```python
from build123d import *

# Parameters (mm, degrees)
SKETCH1_R                       = 62.5
SKETCH1_R_2                     = 36
BOSS_EXTRUDE1_DEPTH             = 5
SKETCH1_4_R                     = 51.5
SKETCH1_4_R_2                   = 36
BOSS_EXTRUDE2_DEPTH             = 14.5
F_4_0MM_DOWEL_HOLE3_D           = 4
F_4_0MM_DOWEL_HOLE3_CSINK_D     = 4.05
F_4_0MM_DOWEL_HOLE3_CSINK_ANGLE = 90
SKETCH11_R                      = 47.5
CUT_EXTRUDE4_DEPTH              = 10.5
FILLET1_R                       = 1


with BuildPart() as part:
    # Sketch1 → Boss-Extrude1 (new body)
    with BuildSketch(Plane.XY):
        Circle(SKETCH1_R)
        Circle(SKETCH1_R_2, mode=Mode.SUBTRACT)
    extrude(amount=BOSS_EXTRUDE1_DEPTH)

    # Sketch1_4 → Boss-Extrude2 (add)
    with BuildSketch(Plane.XY):
        with Locations(Location((0, 0, 0), (0, 0, 180))):
            Circle(SKETCH1_4_R)
        Circle(SKETCH1_4_R_2, mode=Mode.SUBTRACT)
    extrude(amount=BOSS_EXTRUDE2_DEPTH)

    # 4.0mm Dowel Hole3 (through all)
    with Locations(Plane(origin=(0, 0, 0), x_dir=(-1, 0, 0), z_dir=(0, 0, -1))):
        with Locations((0, 57), (0, 42), (40.305086528, 40.305086528), (29.69848481, 29.69848481), (42, 0), (57, 0), (40.305086528, -40.305086528), (29.69848481, -29.69848481), (0, -42), (0, -57), (-29.69848481, -29.69848481), (-40.305086528, -40.305086528), (-42, 0), (-57, 0), (-29.69848481, 29.69848481), (-40.305086528, 40.305086528)):
            CounterSinkHole(F_4_0MM_DOWEL_HOLE3_D / 2, F_4_0MM_DOWEL_HOLE3_CSINK_D / 2, counter_sink_angle=F_4_0MM_DOWEL_HOLE3_CSINK_ANGLE)

    # Sketch11 → Cut-Extrude4 (cut)
    with BuildSketch(Plane.XY):
        with Locations(Location((0, 0, 0), (0, 0, 180))):
            Circle(SKETCH11_R)
    extrude(amount=CUT_EXTRUDE4_DEPTH, mode=Mode.SUBTRACT)

    # Fillet1
    fillet1_edges = [part.edges().sort_by_distance(p)[0] for p in [
        (51.5, 0, 5),
        (51.5, 0, 14.5),
        (47.5, 0, 10.5),
    ]]
    fillet(fillet1_edges, radius=FILLET1_R)


solid = part.part
```
The listing builds one solid part. Answer for the finished solid, in the listing's coordinates (mm). A direction names the side the tool comes from. Round coordinates to 2 decimals unless told otherwise and drop trailing zeros. Loops run counter-clockwise (first coordinate to the right, second up) from the corner with the lowest first, then second, coordinate; pieces in that order, holes last.
Q1. Section A-A, the plane x = 57 is taken. Determine the outline of the cut face in (y, z) (3 decimals), then the cut area to 3 significant figures.
Q2. For a pull along X with two mould halves and no side action, classify faces 1 (the face through (-62.44, 2.75, 2.46)), 2 (the face through (-42, -32, 5)), 3 (the face through (0, 40, 13)) as released by +X, released by -X, zero draft, split by the parting line, or undercut.
Q3. Which of the six approach directions +Z, -Z, +X, -X, +Y, -Y give full straight-line access (tool end or side, diameter ignored) to faces 4 (the face through (-40.565, 42.288, 2.547)), 5 (the face through (35, 10, 10.5))?
Q4. Find the intervals of material crossed by line 1 (Y direction, x = 0, z = 3.3); line 2 (Y direction, x = 0, z = 12.6); line 3 (Z direction, x = 26.5, y = -54.5), in increasing order.
Q5. Section B-B, the plane y = 0 is taken. Count the separate pieces of the cut face and the enclosed holes in it, then the cut area to 3 significant figures.
Q6. Given pin 1 Ø3.5 at (x, y) = (42, 0) entering from -Z; pin 2 Ø8 at (x, z) = (33.5, 6) entering from -Y; pin 3 Ø8 at (x, z) = (-46, 12) entering from -Y; pin 4 Ø5 at (x, y) = (-42, 0) entering from -Z, each flat-ended and moving along its own axis, determine where each tip first touches the part or whether it passes through.
Completed:
1. outline: (-25.637, 0) - (-2.025, 0) - (-2, 0.025) - (-2, 5) - (-25.637, 5) - close; (2, 0.025) - (2.025, 0) - (25.637, 0) - (25.637, 5) - (2, 5) - close
1. area: 236 mm2
2. face 1: split by the parting line
2. face 2: zero draft
2. face 3: undercut
3. face 4: +Z, -Z
3. face 5: -Z
4. line 1: y = -62.5 to -59, -55 to -47.5, 47.5 to 55, 59 to 62.5
4. line 2: y = -51.5 to -44, -40 to -36, 36 to 40, 44 to 51.5
4. line 3: z = 0 to 5
5. separate pieces: 6
5. enclosed holes: 0
5. area: 246 mm2
6. pin 1: passes through
6. pin 2: stops at y = -55.03
6. pin 3: stops at y = -29.8
6. pin 4: stops at z = 10.5
